Drawing for the job (mm, zero at the part's lowest x, y, z). A direction names the side the tool comes from. Coordinates: 2 decimals unless noted, no trailing zeros. Write each loop counter-clockwise with the first axis right and the second up, starting at its lowest first coordinate (ties: lowest second). Pieces come first, ordered by that corner, then holes. Notation, with made-up numbers: (1.25, -39) -> (60.25, -39) arc R11 cw to (60.25, -21) -> close; hole circle Ø9 at (22, 15.5). An arc over 180 degrees is marked (long way). Write each question's results on one line, items separated by ' | '. Start each with the question number.
Q1. Drop a flat-ended pin along its axis: pin 1 Ø1.5 at (y, z) = (28, 75) entering from +X (3 decimals). Give the stop position or say it passes through.
Q2. Drill centre lines: line 1 (Z direction, x = 10.5, y = 45.5) (3 decimals); line 2 (X direction, y = 22.5, z = 46.5) (3 decimals); line 3 (X direction, y = 12, z = 164) (3 decimals). Where is each one in solid material? Low to high.
Q3. Saw through at A-A on y = 12.7. Give the cut face in (x, z) (3 decimals), and give its area (3 significant figures).
Q4. Two-plate mould, pull along Z, no slides. Class the marked faces 1, 2, 3 and 4: released by +Z, released by -Z, zero draft, split by the parting line, or undercut.
Q5. Saw through at D-D on y = 59.5. Give the cut face in (x, z) (3 decimals), and give its area (3 significant figures).
Q6. Tool access for the marked faces 5 and 6: list every direction of +Z, -Z, +X, -X, +Y, -Y with a clear straight run to the whole face (end or side of a thin tool).
Q7. Saw through at B-B on x = 23. Give the cut face in (y, z) (3 decimals).
Q8. Saw through at C-C on x = 36. Give the cut face in (y, z) (3 decimals).
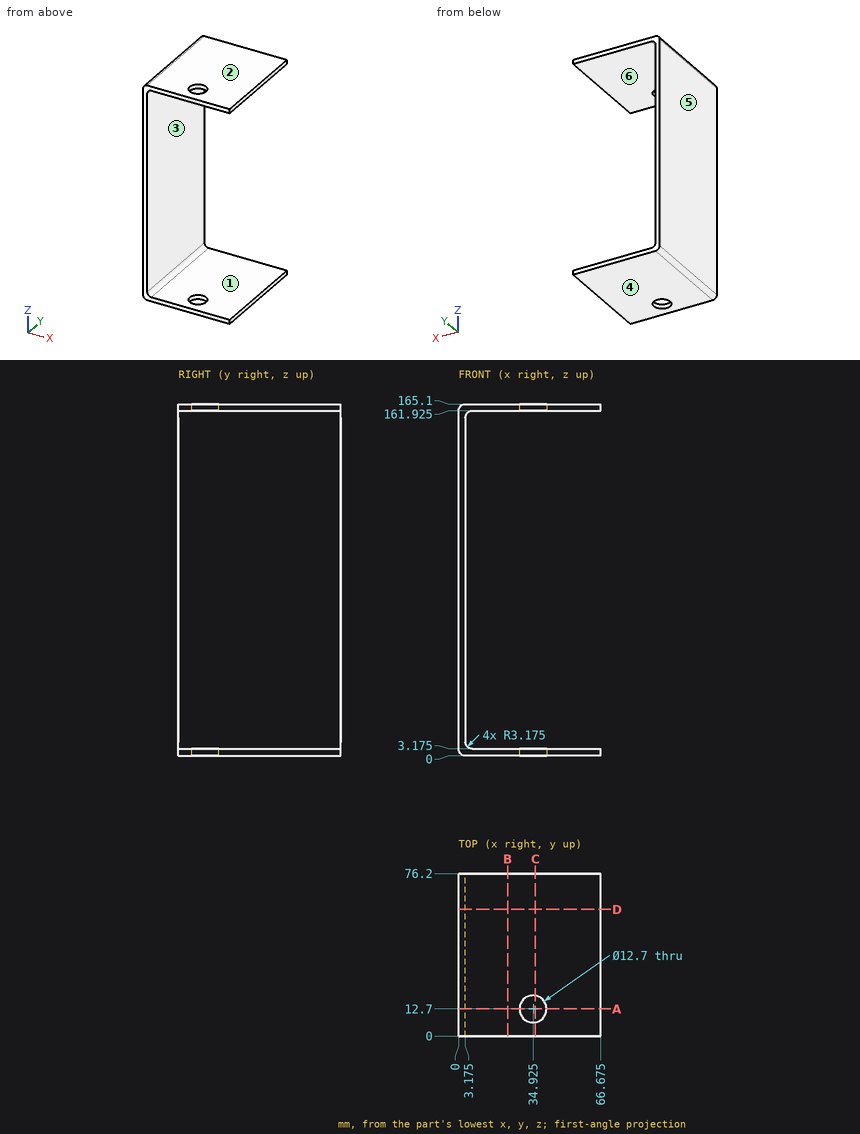
Returned:
1) pin 1: stops at x = 3.175
2) line 1: z = 0 to 3.175, 161.925 to 165.1 | line 2: x = 0 to 3.175 | line 3: x = 0.772 to 28.614, 41.236 to 66.675
3) outline: (0, 3.175) arc R3.175 ccw to (3.175, 0) -> (28.575, 0) -> (28.575, 3.175) -> (6.35, 3.175) arc R3.175 cw to (3.175, 6.35) -> (3.175, 158.75) arc R3.175 cw to (6.35, 161.925) -> (28.575, 161.925) -> (28.575, 165.1) -> (3.175, 165.1) arc R3.175 ccw to (0, 161.925) -> close; (41.275, 0) -> (66.675, 0) -> (66.675, 3.175) -> (41.275, 3.175) -> close; (41.275, 161.925) -> (66.675, 161.925) -> (66.675, 165.1) -> (41.275, 165.1) -> close | area: 847 mm2
4) face 1: undercut | face 2: released by +Z | face 3: undercut | face 4: released by -Z
5) outline: (0, 3.175) arc R3.175 ccw to (3.175, 0) -> (66.675, 0) -> (66.675, 3.175) -> (6.35, 3.175) arc R3.175 cw to (3.175, 6.35) -> (3.175, 158.75) arc R3.175 cw to (6.35, 161.925) -> (66.675, 161.925) -> (66.675, 165.1) -> (3.175, 165.1) arc R3.175 ccw to (0, 161.925) -> close | area: 927 mm2
6) face 5: +Z, -Z, -X, +Y, -Y | face 6: +X, +Y, -Y
7) outline: (0, 0) -> (76.2, 0) -> (76.2, 3.175) -> (0, 3.175) -> close; (0, 161.925) -> (76.2, 161.925) -> (76.2, 165.1) -> (0, 165.1) -> close
8) outline: (0, 0) -> (6.442, 0) -> (6.442, 3.175) -> (0, 3.175) -> close; (0, 161.925) -> (6.442, 161.925) -> (6.442, 165.1) -> (0, 165.1) -> close; (18.958, 0) -> (76.2, 0) -> (76.2, 3.175) -> (18.958, 3.175) -> close; (18.958, 161.925) -> (76.2, 161.925) -> (76.2, 165.1) -> (18.958, 165.1) -> close
